from build123d import *

# Parameters (mm, degrees)
F0_R     = 29.5
F1_DEPTH = 86
F2_R     = 4
F3_DEPTH = 27
F5_W     = 6.35
F5_H     = 9.525
F6_DEPTH = 50.8
F4_R     = 2.25
F7_DEPTH = 25.4


with BuildPart() as f1:
    # F0 (on Front) → F1 (new body)
    with BuildSketch(Plane.XZ):
        Circle(F0_R)
    extrude(amount=F1_DEPTH)

    # F2 (on face) → F3 (join)
    with BuildSketch(Plane.XZ.offset(86)):
        Circle(F2_R)
    extrude(amount=F3_DEPTH)

    # F5 (on Right) → F6 (join)
    with BuildSketch(Plane.YZ):
        with Locations((-82.825, 0)):
            Rectangle(F5_W, F5_H)
    extrude(amount=F6_DEPTH)

    # F4 (on face) → F7 (cut)
    with BuildSketch(Plane.XZ.offset(86)):
        with BuildLine():
            ThreePointArc((9.722718, 9.722718), (12.174746, 9.23498), (13.563708, 11.313708))
            ThreePointArc((13.563708, 11.313708), (10.452671, 13.392437), (9.722718, 9.722718))
        make_face()
        with Locations((-11.313708, 11.313708)):
            Circle(F4_R)
        with Locations((-11.313708, -11.313708)):
            Circle(F4_R)
        with Locations((11.313708, -11.313708)):
            Circle(F4_R)
    extrude(amount=-F7_DEPTH, mode=Mode.SUBTRACT)


solid = f1.part
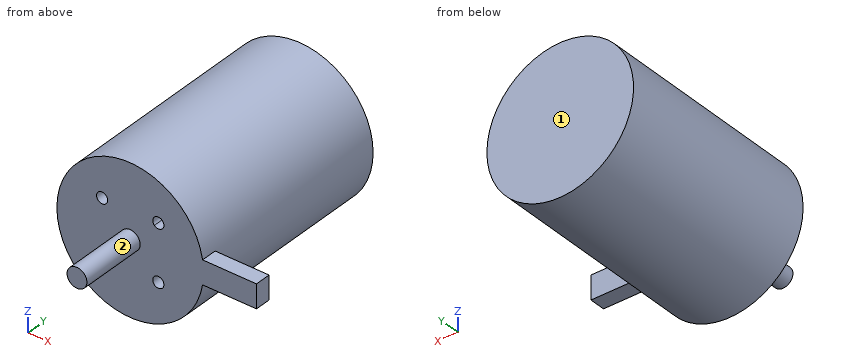
Input: part model. Units: mm. Frame: model coordinates. Face numbers are marked on the shaded views. A direction names the side the tool comes from. Give positions to 0.01 mm unless a question says otherwise; leave off trailing zeros. Write each loop counter-clockwise with the first axis right and the second up, starting at its lowest first coordinate (ties: lowest second). Pieces come first, ordered by that corner, then holes.
Q1. Section A-A, the plane x = 0. Output: boundary loops of the cut face in (y, z).
Q2. Section B-B, the plane z = 0. Output: boundary loops of the cut face in (x, y).
Q3. First-contact query: P1, Ø5, axis at x = 11.31, z = -11.31, coming from the -Y side; P2, Ø2, axis at x = 11.5, z = 11.5, coming from the -Y side; P3, Ø10, axis at x = 31.5, y = -35.5, coming from the +Z side. Flat tips, straight axial feed; report the tip coordinate or a pass-through.
Q4. Material intervals for probe 1 along Y at (x, z) = (13.5, -4); probe 2 along X at (y, z) = (-64.5, 1); probe 3 along Y at (x, z) = (41, 0), sorted ascending.
Q5. Section C-C, the plane y = -62. Output: boundary loops of the cut face in (x, z).
Q6. Section D-D, the plane y = -103. Output: boundary loops of the cut face in (x, z).
Q7. Set-up query: the marked faces 1 and 2. Return all of +Z, -Z, +X, -X, +Y, -Y with unobstructed straight access to the full face (end or side cutting, diameter ignored); none if empty.
Filled in:
1. outline: (-113, -4) - (-86, -4) - (-86, -29.5) - (0, -29.5) - (0, 29.5) - (-86, 29.5) - (-86, 4) - (-113, 4) - close
2. outline: (-29.5, -86) - (-4, -86) - (-4, -113) - (4, -113) - (4, -86) - (50.8, -86) - (50.8, -79.65) - (29.5, -79.65) - (29.5, 0) - (-29.5, 0) - close
3. P1: stops at y = -86
3. P2: stops at y = -60.6
3. P3: stops at z = 12.96
4. probe 1: y = -86 to 0
4. probe 2: x = -29.48 to 29.48
4. probe 3: y = -86 to -79.65
5. outline: circle Ø59 at (0, 0); hole circle Ø4.5 at (-11.31, -11.31); hole circle Ø4.5 at (-11.31, 11.31); hole circle Ø4.5 at (11.31, -11.31); hole circle Ø4.5 at (11.31, 11.31)
6. outline: circle Ø8 at (0, 0)
7. face 1: +Z, -Z, +X, -X, +Y
7. face 2: -Y
